Source: CAD feature listing. Evaluate the final solid. Frame: model axes, mm. A direction names the side the tool comes from. Give positions to 0.01 mm unless a question says otherwise; leave off trailing zeros. Order: outer loops, then holes, each group sorted by start corner. A loop starts at its lowest first (then second) coordinate and runs counter-clockwise, first axis right, second up.
from build123d import *

# Parameters (mm, degrees)
CROQUIS1_R              = 1.75
SALIENTE_EXTRUIR1_DEPTH = 20
REDONDEO1_R             = 20


with BuildPart() as part:
    # Croquis1 → Saliente-Extruir1 (new body)
    with BuildSketch(Plane(origin=(0, 0, 0), x_dir=(1, 0, 0), z_dir=(0, 1, 0))):
        Polygon((-65, 0), (-21.305768696, 0), (30, -55), (65, -55), (65, -75), (21.305768696, -75), (-30, -20), (-65, -20), align=None)
        with Locations(Location((-50, -10, 0), (0, 0, 270))):
            Circle(CROQUIS1_R, mode=Mode.SUBTRACT)
        with Locations(Location((50, -65, 0), (0, 0, 270))):
            Circle(CROQUIS1_R, mode=Mode.SUBTRACT)
    extrude(amount=SALIENTE_EXTRUIR1_DEPTH)

    # Redondeo1
    redondeo1_edges = [part.edges().sort_by_distance(p)[0] for p in [
        (-21.305768696, 10, 0),
        (30, 10, 55),
        (21.305768696, 10, 75),
        (-30, 10, 20),
    ]]
    fillet(redondeo1_edges, radius=REDONDEO1_R)


solid = part.part
1) Section query D-D on x = 10.5. Output: boundary loops of the cut face in (y, z).
Checks:
outline: (0, 34.1) - (20, 34.1) - (20, 63.42) - (0, 63.42) - close
2) Pull-direction query (X, two-part tool) for faces 4 (the face through (-4.07, 9.86, 47.8)), 5 (the face through (65, 10, 65)), 6 (the face through (-51.71, 9.86, 9.62)), 7 (the face through (49.33, 9.86, 66.617)); classes: +X half, -X half, draft (parallel to the pull), parting line (faces both ways), or undercut.
Checks:
face 4: -X half
face 5: +X half
face 6: undercut
face 7: undercut
3) Reachability of faces 1 (the face through (-48, 10, 0)), 2 (the face through (-52, 10, 20)), 3 (the face through (52, 10, 55)) from +Z, -Z, +X, -X, +Y, -Y: full face, straight path, thin tool, end or side. Return the list, or none.
Checks:
face 1: -Z, +X, -X, +Y, -Y
face 2: +Z, -X, +Y, -Y
face 3: -Z, +X, +Y, -Y
4) Section query A-A on x = 50. Output: boundary loops of the cut face in (y, z).
Checks:
outline: (0, 55) - (20, 55) - (20, 63.25) - (0, 63.25) - close; (0, 66.75) - (20, 66.75) - (20, 75) - (0, 75) - close
5) Section query C-C on z = 65. Output: boundary loops of the cut face in (x, y), and give its area (3 significant figures).
Checks:
outline: (11.98, 0) - (48.25, 0) - (48.25, 20) - (11.98, 20) - close; (51.75, 0) - (65, 0) - (65, 20) - (51.75, 20) - close
area: 990 mm2
6) Section query B-B on y = 13.75. Output: boundary loops of the cut face in (x, z), and give its area (3 significant figures).
Checks:
outline: (-65, 0) - (-30, 0) arc R20 ccw to (-15.38, 6.36) - (24.07, 48.64) arc R20 cw to (38.69, 55) - (65, 55) - (65, 75) - (30, 75) arc R20 ccw to (15.38, 68.64) - (-24.07, 26.36) arc R20 cw to (-38.69, 20) - (-65, 20) - close; hole circle Ø3.5 at (-50, 10); hole circle Ø3.5 at (50, 65)
area: 3,060 mm2
7) Ray query, L1, parallel to Z at x = 40, y = 3.5; L2, parallel to X at y = 15.5, z = 65; L3, parallel to X at y = 7, z = 10. Return the intervals inside material, ascending.
Checks:
L1: z = 55 to 75
L2: x = 11.98 to 48.25, 51.75 to 65
L3: x = -65 to -51.75, -48.25 to -11.98
8) First-contact query: pin 1 Ø5.5 at (x, z) = (-50, 10) entering from -Y; pin 2 Ø10 at (x, y) = (50, 6.5) entering from -Z; pin 3 Ø10 at (x, y) = (-19.5, 6) entering from -Z; pin 4 Ø3 at (x, y) = (-13, 6.5) entering from +Z. Flat tips, straight axial feed; report the tip coordinate or a pass-through.
Checks:
pin 1: stops at y = 0
pin 2: stops at z = 55
pin 3: stops at z = 0.77
pin 4: stops at z = 39.83
